For this review, use the dimensioned drawing (mm, ordinates from the lowest corner) and the shaded views. Coordinates: 2 decimals unless noted, no trailing zeros. Loops run counter-clockwise (first coordinate to the right, second up) from the corner with the lowest first, then second, coordinate; pieces in that order, holes last. Notation, with made-up numbers: (-14, 56) - (14, 56) arc R20 cw to (14, 88) - close; hole circle Ø3 at (11.25, -8.75). An arc over 180 degrees is marked (long way). Return JSON: item names as keys, results as strings. Group by question number.
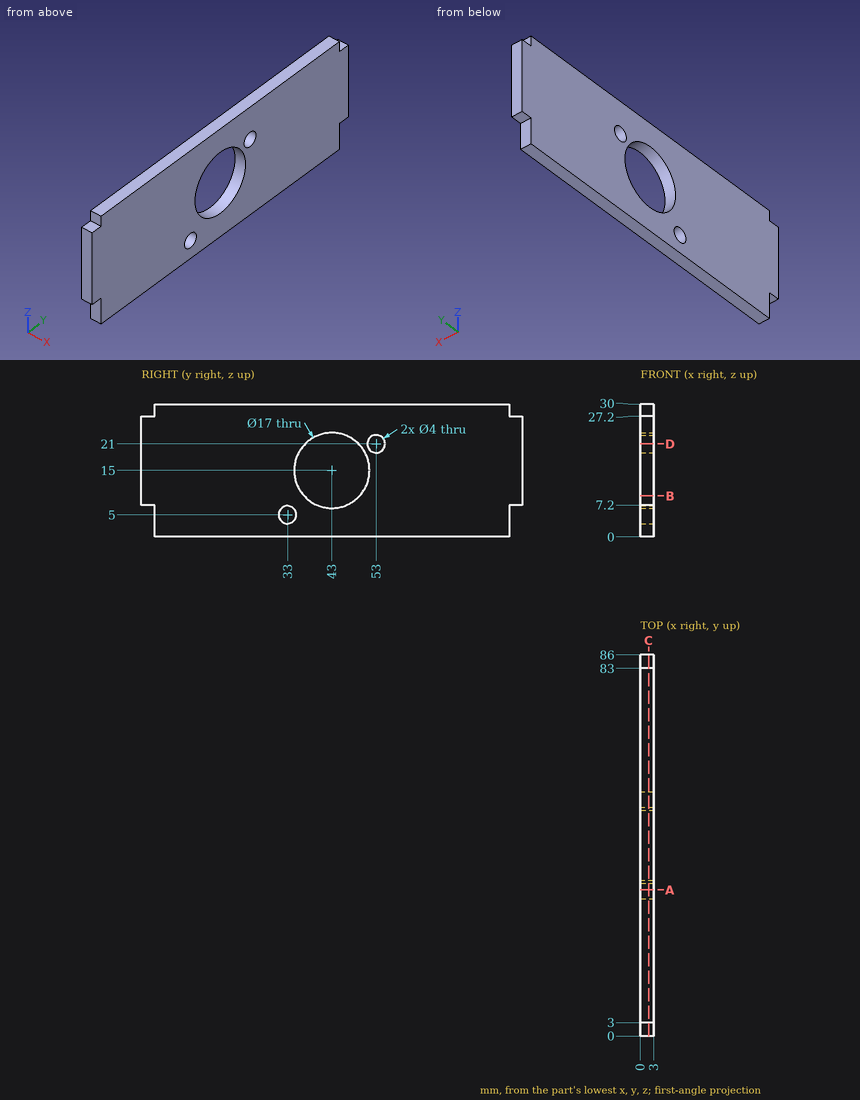
Item 1: To check wall thickness, follow line 1 (Z direction, x = 1.8, y = 53); line 2 (Y direction, x = 2.7, z = 28.5); line 3 (Y direction, x = 2.8, z = 10.25). State the ranges of each line that lie inside material, in increasing order. Write a range as from..to.
Item 2: For P1, Ø1.5, axis at x = 2, z = 5, coming from the -Y side; P2, Ø3, axis at y = 53, z = 21, coming from the +X side; P3, Ø0.8, axis at x = 1.5, z = 29.5, coming from the +Y side; P4, Ø1.5, axis at x = 1.5, y = 2, coming from the -Z side, all flat-tipped, find the tip position at first contact; note any pin that passes through.
Item 3: Add section D-D (z = 21). State the section outline as (x, y) points, then the cut area to 3 significant figures.
Item 4: Add section A-A (y = 33). State the section outline as (x, z) points.
Item 5: Add section C-C (x = 1.85). State the section outline as (y, z) points.
Item 6: Add section B-B (z = 9.25). State the section outline as (x, y) points, then the cut area to 3 significant figures.
Answers below:
{
 "1": {"line 1": "z = 0..19, 23..30", "line 2": "y = 3..83", "line 3": "y = 0..35.95, 50.05..86"},
 "2": {"P1": "stops at y = 3", "P2": "passes through", "P3": "stops at y = 83", "P4": "stops at z = 7.2"},
 "3": {"outline": "(0, 0) - (3, 0) - (3, 36.98) - (0, 36.98) - close; (0, 49.02) - (3, 49.02) - (3, 51) - (0, 51) - close; (0, 55) - (3, 55) - (3, 86) - (0, 86) - close", "area": "210 mm^2"},
 "4": {"outline": "(0, 0) - (3, 0) - (3, 3) - (0, 3) - close; (0, 7) - (3, 7) - (3, 30) - (0, 30) - close"},
 "5": {"outline": "(0, 7.2) - (3, 7.2) - (3, 0) - (83, 0) - (83, 7.2) - (86, 7.2) - (86, 27.2) - (83, 27.2) - (83, 30) - (3, 30) - (3, 27.2) - (0, 27.2) - close; hole circle Ø4 at (33, 5); hole circle Ø17 at (43, 15); hole circle Ø4 at (53, 21)"},
 "6": {"outline": "(0, 0) - (3, 0) - (3, 36.74) - (0, 36.74) - close; (0, 49.26) - (3, 49.26) - (3, 86) - (0, 86) - close", "area": "220 mm^2"}
}
